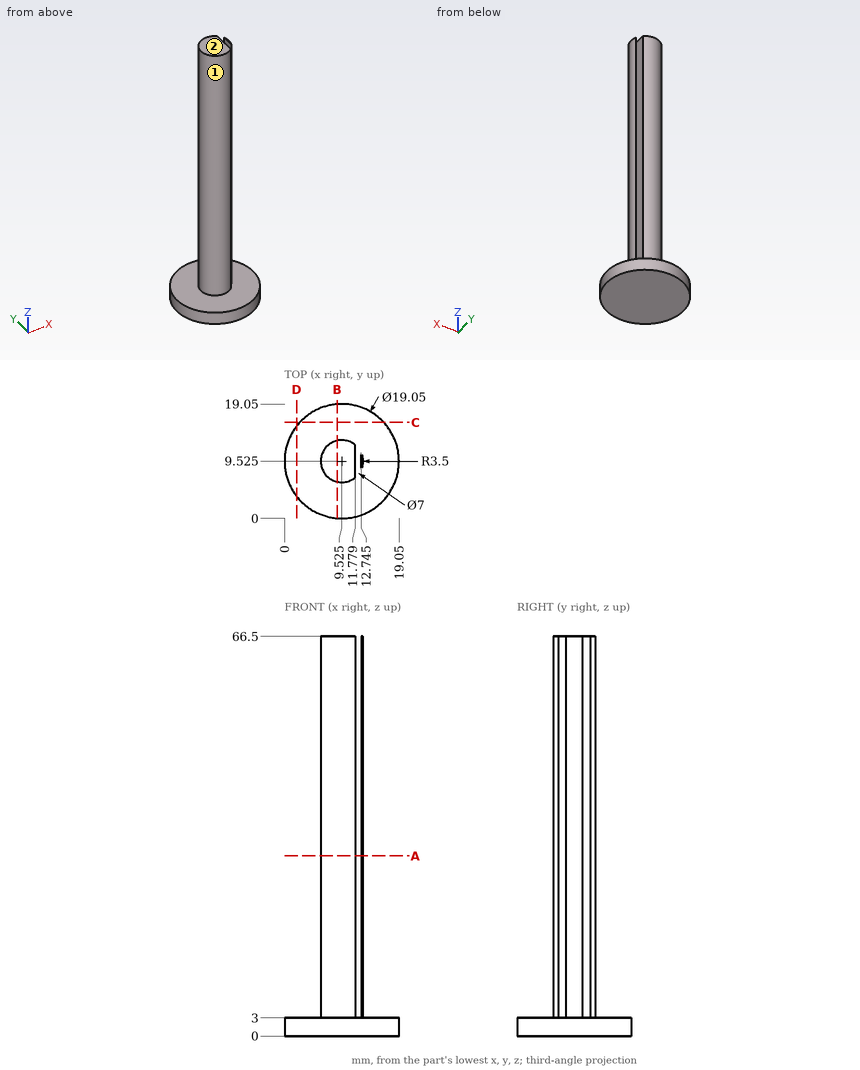
Drawing for the job (mm, zero at the part's lowest x, y, z). A direction names the side the tool comes from. Give positions to 0.01 mm unless a question says otherwise; leave off trailing zeros. Loops run counter-clockwise (first coordinate to the right, second up) from the corner with the lowest first, then second, coordinate; pieces in that order, holes last.
Item 1: Slice it at A-A (z = 30). Write the cut outline in (x, y) (1 decimal).
Check values:
outline: (11.8, 6.8) - (11.8, 12.2) arc R3.5 ccw (long way) to start; (12.7, 8.2) arc R3.5 ccw to (12.7, 10.9) - close
Item 2: Which spindle directions (+Z, -Z, +X, -X, +Y, -Y) get a long thin tool onto all of the face, cutting with end or side? Do the marked faces 1 and 2. Say none if no direction does.
Check values:
face 1: +Z
face 2: +Z, +X, -X, +Y, -Y
Item 3: Slice it at B-B (x = 8.75). Write the cut outline in (y, z).
Check values:
outline: (0.03, 0) - (19.02, 0) - (19.02, 3) - (12.94, 3) - (12.94, 66.5) - (6.11, 66.5) - (6.11, 3) - (0.03, 3) - close
Item 4: Drill centre lines: line 1 along Z through (x, y) = (17, 5.5); line 2 along Y through (x, z) = (11.5, 14.5) (1 decimal); line 3 along Y through (x, z) = (7.25, 43) (1 decimal). Where is each one in solid material? Low to high.
Check values:
line 1: z = 0 to 3
line 2: y = 6.6 to 12.4
line 3: y = 6.9 to 12.2
Item 5: Slice it at D-D (x = 2). Write the cut outline in (y, z) (1 decimal).
Check values:
outline: (3.7, 0) - (15.4, 0) - (15.4, 3) - (3.7, 3) - close
Item 6: Drop flat-ended pins along their axis: P1, Ø1, axis at x = 3, y = 15, coming from the -Z side; P2, Ø6, axis at x = 7.5, z = 39, coming from the -Y side (3 decimals); P3, Ø1.5, axis at x = 8, z = 30, coming from the -Y side; P4, Ø1.6, axis at y = 8, z = 35.5, coming from the +X side. Give the stop position or say it passes through.
Check values:
P1: stops at z = 0
P2: stops at y = 6.025
P3: stops at y = 6.11
P4: stops at x = 12.95
Item 7: Slice it at C-C (y = 16). Write the cut outline in (x, z), plus the area to 3 significant figures.
Check values:
outline: (2.54, 0) - (16.51, 0) - (16.51, 3) - (2.54, 3) - close
area: 41.9 mm2
